Can you work these out from the drawing? Everything is in mm from the part's minimum corner. Give positions to 0.01 mm unless a question says otherwise; leave off trailing zeros. Loops run counter-clockwise (first coordinate to the right, second up) from the corner with the lowest first, then second, coordinate; pieces in that order, holes last.
Q1. I need wall thicknesses on line 1 (Z direction, x = 7, y = 3.5); line 2 (Z direction, x = 22.5, y = 6.25); line 3 (Z direction, x = 24, y = 6.75). Which ranges of each line are inside material? Lowest first, please.
Q2. If we section it at C-C (z = 45.5): Please give me the cut outline in (x, y).
Q3. If we section it at A-A (x = 22.5): Please give me the cut outline in (y, z).
Q4. If we section it at B-B (z = 55): Please give me the cut outline in (x, y), plus the area to 3 significant figures.
Q5. Will this pin go through, and if not, where does the flat tip stop? P1, Ø12, axis at x = 22.5, z = 30, coming from the +Y side.
Q6. If we section it at D-D (y = 3): Please give me the cut outline in (x, z), plus the area to 3 significant figures.
Q7. We'd pull the mould along X, two halves only. Please class the marked faces 1, 2 and 3: +X half, -X half, draft (parallel to the pull), parting line (faces both ways), or undercut.
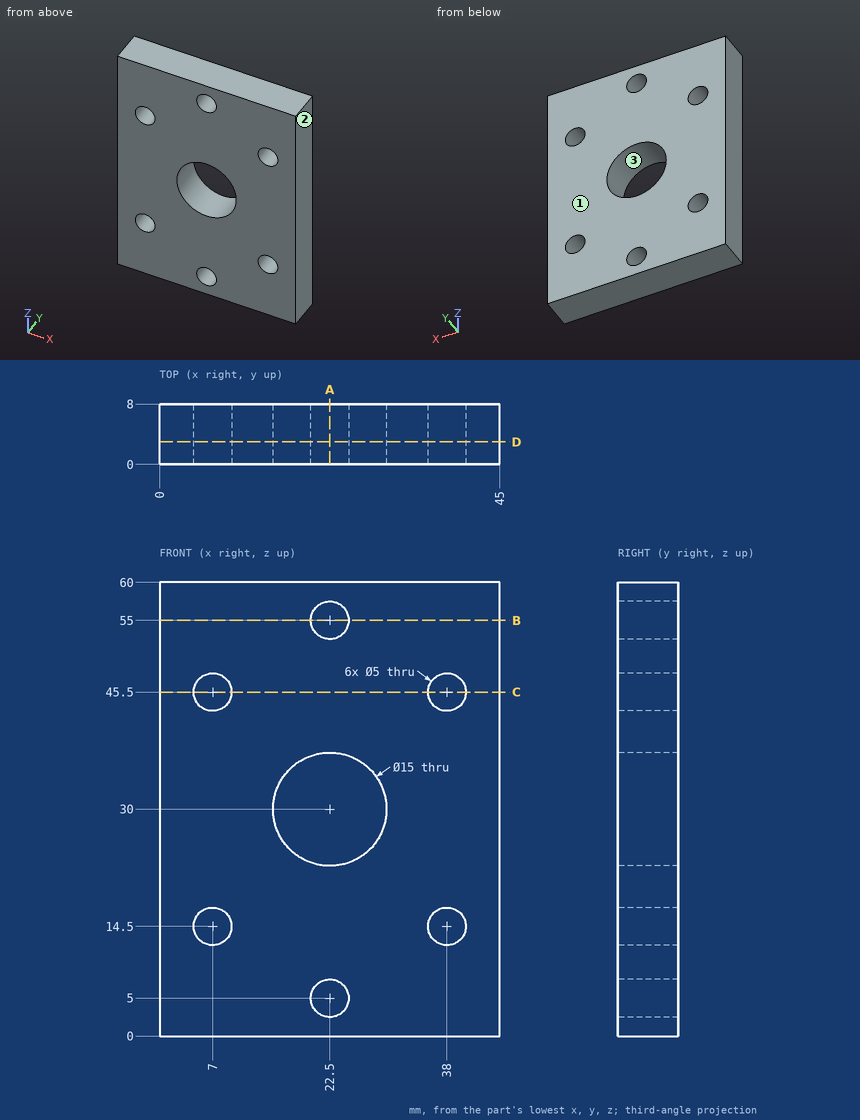
Check sheet entries:
1. line 1: z = 0 to 12, 17 to 43, 48 to 60
1. line 2: z = 0 to 2.5, 7.5 to 22.5, 37.5 to 52.5, 57.5 to 60
1. line 3: z = 0 to 3, 7 to 22.65, 37.35 to 53, 57 to 60
2. outline: (0, 0) - (4.5, 0) - (4.5, 8) - (0, 8) - close; (9.5, 0) - (35.5, 0) - (35.5, 8) - (9.5, 8) - close; (40.5, 0) - (45, 0) - (45, 8) - (40.5, 8) - close
3. outline: (0, 0) - (8, 0) - (8, 2.5) - (0, 2.5) - close; (0, 7.5) - (8, 7.5) - (8, 22.5) - (0, 22.5) - close; (0, 37.5) - (8, 37.5) - (8, 52.5) - (0, 52.5) - close; (0, 57.5) - (8, 57.5) - (8, 60) - (0, 60) - close
4. outline: (0, 0) - (20, 0) - (20, 8) - (0, 8) - close; (25, 0) - (45, 0) - (45, 8) - (25, 8) - close
4. area: 320 mm2
5. P1: passes through
6. outline: (0, 0) - (45, 0) - (45, 60) - (0, 60) - close; hole circle Ø5 at (7, 14.5); hole circle Ø5 at (7, 45.5); hole circle Ø15 at (22.5, 30); hole circle Ø5 at (22.5, 5); hole circle Ø5 at (22.5, 55); hole circle Ø5 at (38, 14.5); hole circle Ø5 at (38, 45.5)
6. area: 2,410 mm2
7. face 1: draft
7. face 2: +X half
7. face 3: undercut
